```python
from build123d import *

# Parameters (mm, degrees)
EXTRUDE_1_DEPTH     = 3.4
SKETCH_2_W          = 0.4
SKETCH_2_H          = 3
CUT_EXTRUDE_1_DEPTH = 7.83637537


with BuildPart() as part:
    # Эскиз1 → Бобышка-Вытянуть1 (new body)
    with BuildSketch(Plane(origin=(0, 0, 0), x_dir=(1, 0, 0), z_dir=(0, 1, 0))):
        Polygon((2.37904421, -4), (-2.37904421, -4), (-4.37904421, -4), (-4.37904421, 0), (-2.37904421, 0), (-2.37904421, 3), (2.37904421, 3), (2.37904421, 0), (4.37904421, 0), (4.37904421, -4), align=None)
    extrude(amount=EXTRUDE_1_DEPTH)

    # Эскиз2 → Вырез-Вытянуть1 (cut, through all)
    with BuildSketch(Plane(origin=(0, 0, 0), x_dir=(1, 0, 0), z_dir=(0, 1, 0))):
        with Locations((2.37904421, 1.5)):
            Rectangle(SKETCH_2_W, SKETCH_2_H)
        with Locations((-2.37904421, 1.5)):
            Rectangle(SKETCH_2_W, SKETCH_2_H)
    extrude(amount=CUT_EXTRUDE_1_DEPTH, mode=Mode.SUBTRACT)


solid = part.part
```
Verification items for the finished model (mm, model axes). A direction names the side the tool comes from. Coordinates: 2 decimals unless noted, no trailing zeros. Order: outer loops, then holes, each group sorted by start corner. A loop starts at its lowest first (then second) coordinate and runs counter-clockwise, first axis right, second up. Notation, with made-up numbers: (12, 15) - (24, 15) arc R20 ccw to (24, 54) - close; hole circle Ø9 at (77, 24.25). An arc over 180 degrees is marked (long way). Return JSON: item names as keys, results as strings.
(1) Section check A-A, the plane y = 3.15. Record the cut outline in (x, z), and give its area (3 significant figures).
Filled sheet:
{"outline": "(-4.38, 0) - (-2.18, 0) - (-2.18, -3) - (2.18, -3) - (2.18, 0) - (4.38, 0) - (4.38, 4) - (-4.38, 4) - close", "area": "48.1 mm^2"}
(2) Section check C-C, the plane z = -0.5. Record the cut outline in (x, y), and give its area (3 significant figures).
Filled sheet:
{"outline": "(-2.18, 0) - (2.18, 0) - (2.18, 3.4) - (-2.18, 3.4) - close", "area": "14.8 mm^2"}
(3) Section check B-B, the plane x = 2.75. Record the cut outline in (y, z).
Filled sheet:
{"outline": "(0, 0) - (3.4, 0) - (3.4, 4) - (0, 4) - close"}
(4) Access from +Z, -Z, +X, -X, +Y, -Y to the whole of each face (thin tool, end or side, straight path). Record for faces 1 (the flat face through (0, 3.4, 1)), 2 (the flat face through (-3, 2, 0)), 3 (the flat face through (2.179, 2, -1)).
Filled sheet:
{"face 1": "+Z, -Z, +X, -X, +Y", "face 2": "-Z, -X, +Y, -Y", "face 3": "-Z, +X, +Y, -Y"}
(5) Go/stop test with flat-tipped pins: pin 1 (0.7 mm diameter, centred on x = -3.5, y = 1.5, fed in from -Z); pin 2 (0.9 mm diameter, centred on y = 1.5, z = -1.5, fed in from -X). Record where each tip stops, or that it passes through.
Filled sheet:
{"pin 1": "stops at z = 0", "pin 2": "stops at x = -2.18"}
(6) Thickness scan on line 1 along Z through (x, y) = (2.5, 0.6); line 2 along X through (y, z) = (2.55, -2.5). Record the ranges inside material, lowest first.
Filled sheet:
{"line 1": "z = 0 to 4", "line 2": "x = -2.18 to 2.18"}
